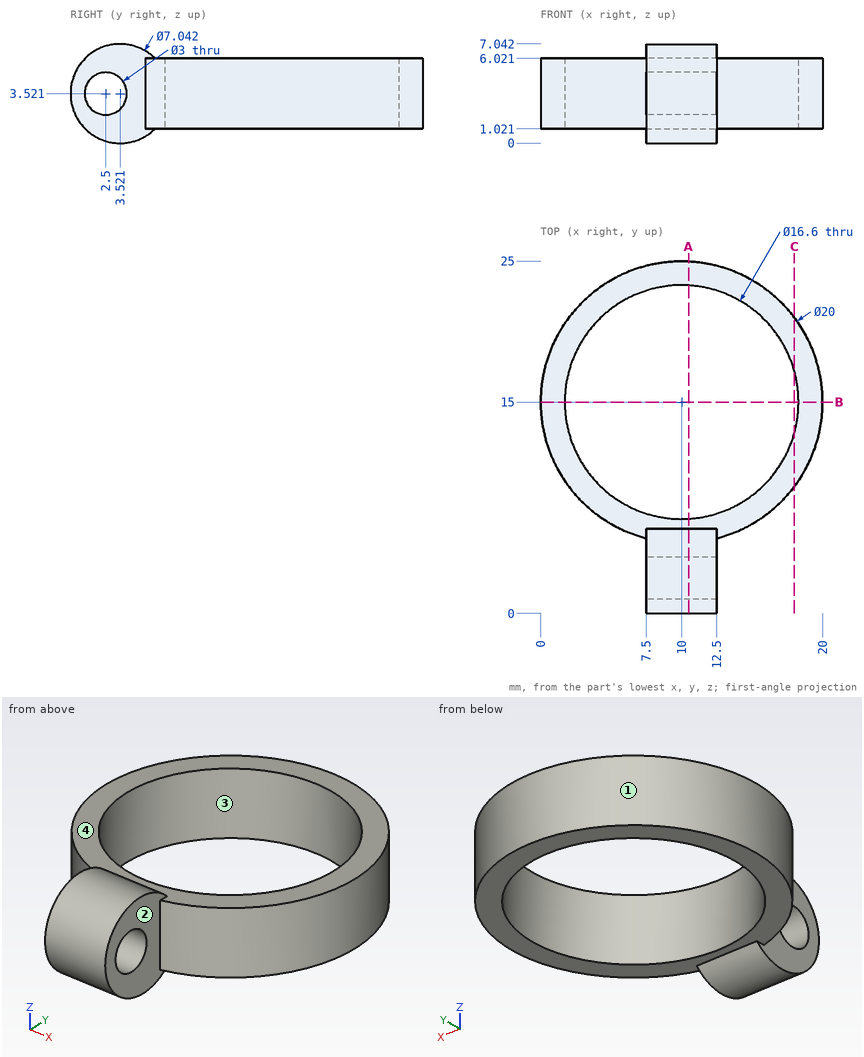
Here's the drawing with two shaded views (mm, measured from the low corner). I have some questions. Give positions to 0.01 mm unless a question says otherwise; leave off trailing zeros. Loops run counter-clockwise (first coordinate to the right, second up) from the corner with the lowest first, then second, coordinate; pieces in that order, holes last. Notation, with made-up numbers: M 6,65.25 L 49,65.25 A16 cw 49,70.25 Z; hole C 71,-22.75 d4. An arc over 180 degrees is marked long. One line per item, written item: value.
(1) Suppose I cut it at C-C on x = 18. List the corners of the cut face in (y, z) for me.
Returned:
outline: M 9,1.02 L 12.79,1.02 L 12.79,6.02 L 9,6.02 Z; M 17.21,1.02 L 21,1.02 L 21,6.02 L 17.21,6.02 Z
(2) Suppose I cut it at A-A on x = 10.5. List the corners of the cut face in (y, z) for me (1 decimal).
Returned:
outline: M 6,1 L 6.7,1 L 6.7,6 L 6,6 A3.5 ccw long Z; M 23.3,1 L 25,1 L 25,6 L 23.3,6 Z; hole C 2.5,3.5 d3
(3) We'd pull the mould along X, two halves only. Please class the marked faces 1, 2, 3 and 4: released by +X, released by -X, zero draft, split by the parting line, or undercut.
Returned:
face 1: split by the parting line
face 2: released by +X
face 3: undercut
face 4: zero draft
(4) Suppose I cut it at B-B on y = 15. List the corners of the cut face in (x, z) for me, plus the area to 3 significant figures.
Returned:
outline: M 0,1.02 L 1.7,1.02 L 1.7,6.02 L 0,6.02 Z; M 18.3,1.02 L 20,1.02 L 20,6.02 L 18.3,6.02 Z
area: 17.0 mm^2
(5) Will these pins go through, and if not, where does the flat tip stop? pin 1 (3 mm diameter, centred on x = 17.5, y = 9, fed in from +Z); pin 2 (1.5 mm diameter, centred on y = 2.5, z = 6, fed in from -X); pin 3 (1 mm diameter, centred on x = 17, y = 13, fed in from +Z); pin 4 (1.5 mm diameter, centred on y = 13.5, z = 4, fed in from +X).
Returned:
pin 1: z = 6.02
pin 2: x = 7.5
pin 3: through
pin 4: x = 19.97
(6) I need wall thicknesses on line 1 (Y direction, x = 10, z = 2.35); line 2 (Y direction, x = 10, z = 2.85) (1 decimal); line 3 (X direction, y = 20, z = 3.25) (1 decimal). Which ranges of each line are inside material? Lowest first, please.
Returned:
line 1: 0.2 to 1.56, 3.44 to 6.7, 23.3 to 25
line 2: 0.1 to 1.2, 3.8 to 6.7, 23.3 to 25
line 3: 1.3 to 3.4, 16.6 to 18.7
